Here's the drawing with two shaded views (mm, measured from the low corner). I have some questions. A direction names the side the tool comes from. Give positions to 0.01 mm unless a question says otherwise; leave off trailing zeros. Loops run counter-clockwise (first coordinate to the right, second up) from the corner with the lowest first, then second, coordinate; pieces in that order, holes last.
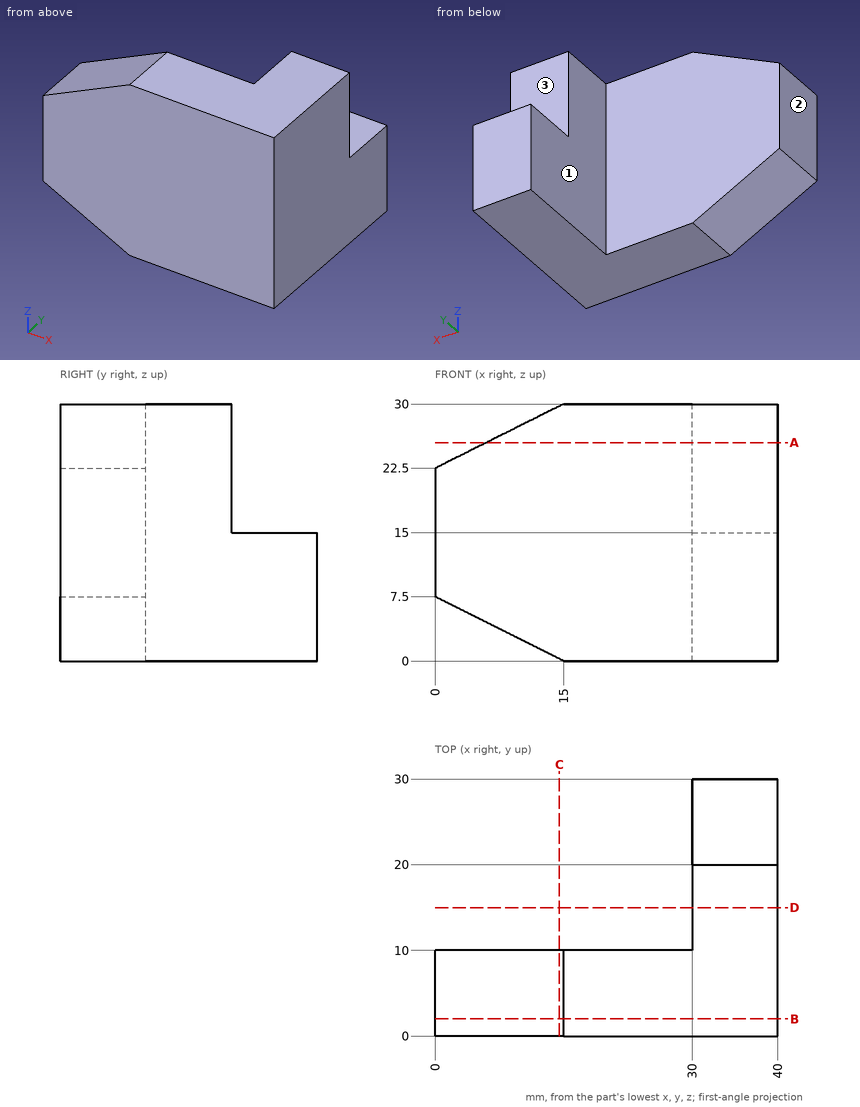
(1) Which directions (+Z, -Z, +X, -X, +Y, -Y) give clear straight access to the entire face, cutting with the end or side of a thin tool? Please do the marked faces 1, 2 and 3.
Returned:
face 1: +Z, -Z, -X, +Y
face 2: +Z, -Z, -X, +Y, -Y
face 3: +Z, +X, -X, +Y
(2) Suppose I cut it at B-B on y = 2. List the corners of the cut face in (x, z) for me, plus the area to 3 significant figures.
Returned:
outline: (0, 7.5) - (15, 0) - (40, 0) - (40, 30) - (15, 30) - (0, 22.5) - close
area: 1,090 mm2
(3) Will these pins go through, and if not, where does the flat tip stop? P1, Ø10, axis at x = 8.5, z = 18, coming from the +Y side; P2, Ø8, axis at x = 37, z = 26, coming from the +Y side; P3, Ø6, axis at y = 15, z = 16, coming from the -X side.
Returned:
P1: stops at y = 10
P2: stops at y = 20
P3: stops at x = 30
(4) Suppose I cut it at A-A on z = 25.5. List the corners of the cut face in (x, y) for me.
Returned:
outline: (6, 0) - (40, 0) - (40, 20) - (30, 20) - (30, 10) - (6, 10) - close
(5) Please list where these lines run through material, in increasing order: probe 1 along X at (y, z) = (19.75, 10.25); probe 2 along Y at (x, z) = (19.5, 10.5); probe 3 along Y at (x, z) = (38, 26.75).
Returned:
probe 1: x = 30 to 40
probe 2: y = 0 to 10
probe 3: y = 0 to 20
(6) Suppose I cut it at D-D on y = 15. List the corners of the cut face in (x, z) for me.
Returned:
outline: (30, 0) - (40, 0) - (40, 30) - (30, 30) - close
(7) Suppose I cut it at C-C on x = 14.5. List the corners of the cut face in (y, z) for me, plus the area to 3 significant figures.
Returned:
outline: (0, 0.25) - (10, 0.25) - (10, 29.75) - (0, 29.75) - close
area: 295 mm2
